Read the model definition and answer for the solid it produces. Units are mm, in the model's axes. Coordinates: 2 decimals unless noted, no trailing zeros. Write each loop counter-clockwise with the first axis right and the second up, starting at its lowest first coordinate (ties: lowest second). Pieces come first, ordered by that corner, then holes. Notation, with made-up numbers: (-12, 27.5) - (41, 27.5) arc R12 cw to (41, 41.5) - close; hole circle Ø11 at (58, -16.75). An arc over 180 degrees is marked (long way). Return JSON: item names as keys, results as strings.
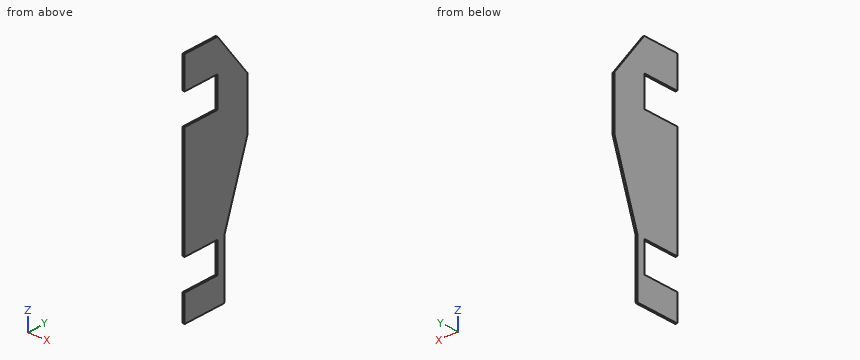
```python
from build123d import *

# Parameters (mm, degrees)
SKETCH1_W           = 620
SKETCH1_H           = 190
BOSS_EXTRUDE1_DEPTH = 5
SKETCH2_W           = 82
SKETCH2_H           = 100
CUT_EXTRUDE1_DEPTH  = 5
FILLET1_R           = 2


with BuildPart() as part:
    # Sketch1 → Boss-Extrude1 (new body)
    with BuildSketch(Plane(origin=(0, 0, 0), x_dir=(0, 0, -1), z_dir=(1, 0, 0))):
        Rectangle(SKETCH1_W, SKETCH1_H)
    extrude(amount=BOSS_EXTRUDE1_DEPTH)

    # Sketch2 → Cut-Extrude1 (cut)
    with BuildSketch(Plane(origin=(5, 0, 0), x_dir=(0, 0, -1), z_dir=(1, 0, 0))):
        Polygon((-310, 95), (-310, 5), (-190, 95), align=None)
        Polygon((310, 95), (-50, 95), (155, 25), (310, 25), align=None)
        with Locations((-183, -45)):
            Rectangle(SKETCH2_W, SKETCH2_H)
        with Locations((197, -45)):
            Rectangle(SKETCH2_W, SKETCH2_H)
    extrude(amount=-CUT_EXTRUDE1_DEPTH, mode=Mode.SUBTRACT)

    # Fillet1
    fillet1_edges = [part.edges().sort_by_distance(p)[0] for p in [
        (2.5, 25, -155),
        (2.5, 95, 50),
        (2.5, 25, -310),
        (2.5, -95, 142),
        (2.5, -95, 224),
        (2.5, -95, -238),
        (2.5, -95, -156),
        (2.5, 5, 310),
        (2.5, 95, 190),
        (2.5, -95, -310),
        (2.5, -95, 310),
    ]]
    fillet(fillet1_edges, radius=FILLET1_R)


solid = part.part
```
(1) A cutting plane is placed at B-B (x = 4.25). Determine the outline of the cut face in (y, z), and give its area (3 significant figures).
Answer:
{"outline": "(-95, -308) arc R2 ccw to (-93, -310) - (23, -310) arc R2 ccw to (25, -308) - (25, -155.33) arc R2 cw to (25.11, -154.69) - (94.89, 49.69) arc R2 ccw to (95, 50.33) - (95, 189.33) arc R2 ccw to (94.6, 190.53) - (5.6, 309.2) arc R2 ccw to (4, 310) - (-93, 310) arc R2 ccw to (-95, 308) - (-95, 226) arc R2 ccw to (-93, 224) - (5, 224) - (5, 142) - (-93, 142) arc R2 ccw to (-95, 140) - (-95, -154) arc R2 ccw to (-93, -156) - (5, -156) - (5, -238) - (-93, -238) arc R2 ccw to (-95, -240) - close", "area": "78,000 mm²"}
(2) A cutting plane is placed at A-A (y = -7.5). Determine the outline of the cut face in (x, z), and give its area (3 significant figures).
Answer:
{"outline": "(0, -310) - (5, -310) - (5, -238) - (0, -238) - close; (0, -156) - (5, -156) - (5, 142) - (0, 142) - close; (0, 224) - (5, 224) - (5, 310) - (0, 310) - close", "area": "2,280 mm²"}
(3) A cutting plane is placed at C-C (z = -25). Determine the outline of the cut face in (x, y).
Answer:
{"outline": "(0, -95) - (5, -95) - (5, 69.39) - (0, 69.39) - close"}
(4) A cutting plane is placed at D-D (y = 47.5). Determine the outline of the cut face in (x, z).
Answer:
{"outline": "(0, -89.11) - (5, -89.11) - (5, 253.33) - (0, 253.33) - close"}
(5) Straight lines are drawn through the part: line 1 (Z direction, x = 2.05, y = -9); line 2 (Y direction, x = 4, z = -254.5); line 3 (Y direction, x = 0.9, z = -180). For each, find the intervals that lie inside material, in ascending order. Write a range as from..to.
Answer:
{"line 1": "-310..-238, -156..142, 224..310", "line 2": "-95..25", "line 3": "5..25"}
(6) Flat-ended cylindrical pins translate along their axes: P1, Ø1.5, axis at x = 3.5, z = -231, coming from the +Y side; P2, Ø1.5, axis at x = 3.5, z = -199.5, coming from the -Y side. Find the tip coordinate at first contact, or state that the pin passes through.
Answer:
{"P1": "y = 25", "P2": "y = 5"}
